Design review of the part built by this model. Coordinates are the model's own, in mm. Round coordinates to 2 decimals unless told otherwise and drop trailing zeros. Write each loop counter-clockwise with the first axis right and the second up, starting at its lowest first coordinate (ties: lowest second). Pieces come first, ordered by that corner, then holes. Notation, with made-up numbers: (-12.75, 55.5) -> (1.25, 55.5) arc R20 cw to (1.25, 73.5) -> close; hole circle Ø3 at (12.5, 23). An arc over 180 degrees is marked (long way). Write item = value, one per line. Start each with the question number.
Item 1: To check wall thickness, follow L1, parallel to X at y = 2.7, z = -10; L2, parallel to Z at x = 67, y = 2.55; L3, parallel to Z at x = 19, y = 3.2. State the ranges of each line that lie inside material, in increasing order.
Item 2: Add section C-C, the plane z = -10. State the section outline as (x, y) points.
Item 3: Add section A-A, the plane x = 7. State the section outline as (y, z) points, then the cut area to 3 significant figures.
Item 4: Add section B-B, the plane y = 3.3. State the section outline as (x, z) points, then the cut area to 3 significant figures.
Item 5: Add section D-D, the plane x = 19. State the section outline as (y, z) points.
Item 6: For pin 1 Ø5 at (x, z) = (19, -10) entering from -Y; pin 2 Ø8 at (x, z) = (63, -18) entering from -Y; pin 3 Ø3 at (y, z) = (4, -17.5) entering from -X, all flat-tipped, find the tip position at first contact; note any pin that passes through.
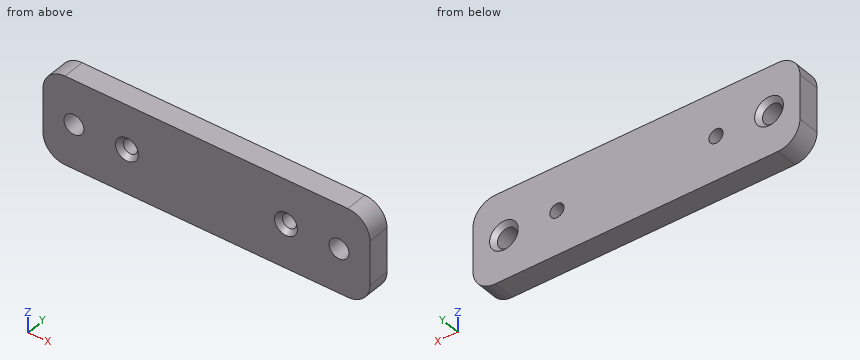
from build123d import *

# Parameters (mm, degrees)
SKETCH_1_W      = 74
SKETCH_1_H      = 20
SKETCH_1_R      = 1.6
SKETCH_1_R_2    = 2.25
EXTRUDE_1_DEPTH = 5
FILLET_2_R      = 5
CHAMFER_1_SIZE  = 1
CHAMFER_2_SIZE  = 1


with BuildPart() as part:
    # Эскиз1 → Бобышка-Вытянуть1 (new body)
    with BuildSketch(Plane(origin=(0, 0, 0), x_dir=(1, 0, 0), z_dir=(0, 1, 0))):
        with Locations((37, 10)):
            Rectangle(SKETCH_1_W, SKETCH_1_H)
        with Locations((19, 10)):
            Circle(SKETCH_1_R, mode=Mode.SUBTRACT)
        with Locations((55, 10)):
            Circle(SKETCH_1_R, mode=Mode.SUBTRACT)
        with Locations((7, 10)):
            Circle(SKETCH_1_R_2, mode=Mode.SUBTRACT)
        with Locations((67, 10)):
            Circle(SKETCH_1_R_2, mode=Mode.SUBTRACT)
    extrude(amount=EXTRUDE_1_DEPTH)

    # Скругление2
    fillet_2_edges = [part.edges().sort_by_distance(p)[0] for p in [
        (0, 2.5, -20),
        (74, 2.5, -20),
        (74, 2.5, 0),
        (0, 2.5, 0),
    ]]
    fillet(fillet_2_edges, radius=FILLET_2_R)

    # Фаска1
    chamfer_1_edges = [part.edges().sort_by_distance(p)[0] for p in [
        (4.75, 5, -10),
        (64.75, 5, -10),
    ]]
    chamfer(chamfer_1_edges, length=CHAMFER_1_SIZE)

    # Фаска2
    chamfer_2_edges = [part.edges().sort_by_distance(p)[0] for p in [
        (17.4, 0, -10),
        (53.4, 0, -10),
    ]]
    chamfer(chamfer_2_edges, length=CHAMFER_2_SIZE)


solid = part.part
Result set:
q1.L1 = 0 to 4.75, 9.25 to 17.4, 20.6 to 53.4, 56.6 to 64.75, 69.25 to 74
q1.L2 = -20 to -12.25, -7.75 to 0
q1.L3 = -20 to -11.6, -8.4 to 0
q2.outline = (0, 0) -> (4.75, 0) -> (4.75, 4) -> (3.75, 5) -> (0, 5) -> close; (9.25, 0) -> (16.4, 0) -> (17.4, 1) -> (17.4, 5) -> (10.25, 5) -> (9.25, 4) -> close; (20.6, 1) -> (21.6, 0) -> (52.4, 0) -> (53.4, 1) -> (53.4, 5) -> (20.6, 5) -> close; (56.6, 1) -> (57.6, 0) -> (64.75, 0) -> (64.75, 4) -> (63.75, 5) -> (56.6, 5) -> close; (69.25, 0) -> (74, 0) -> (74, 5) -> (70.25, 5) -> (69.25, 4) -> close
q3.outline = (0, -20) -> (5, -20) -> (5, -13.25) -> (4, -12.25) -> (0, -12.25) -> close; (0, -7.75) -> (4, -7.75) -> (5, -6.75) -> (5, 0) -> (0, 0) -> close
q3.area = 76.5 mm²
q4.outline = (0, -15) arc R5 ccw to (5, -20) -> (69, -20) arc R5 ccw to (74, -15) -> (74, -5) arc R5 ccw to (69, 0) -> (5, 0) arc R5 ccw to (0, -5) -> close; hole circle Ø4.5 at (7, -10); hole circle Ø3.2 at (19, -10); hole circle Ø3.2 at (55, -10); hole circle Ø4.5 at (67, -10)
q4.area = 1,410 mm²
q5.outline = (0, -20) -> (5, -20) -> (5, -11.6) -> (1, -11.6) -> (0, -12.6) -> close; (0, -7.4) -> (1, -8.4) -> (5, -8.4) -> (5, 0) -> (0, 0) -> close
q6.pin_1 = 0.1
q6.pin_2 = 0
q6.pin_3 = 0.1
